Can you work these out from the drawing? Everything is in mm from the part's minimum corner. A direction names the side the tool comes from. Coordinates: 2 decimals unless noted, no trailing zeros. Order: outer loops, then holes, each group sorted by start corner. A loop starts at its lowest first (then second) coordinate and runs counter-clockwise, first axis right, second up. Notation, with made-up numbers: (-37.5, 69.5) -> (-22.5, 69.5) arc R7 cw to (-22.5, 78.5) -> close; hole circle Ø8 at (64.5, 50). An arc over 180 degrees is marked (long way). Return JSON: item names as keys, results as strings. Group by question number.
1) If we section it at A-A, the plane z = 19.5: Please give me the cut outline in (x, y).
2) For the marked faces 1 and 2, which set-ups out of +Z, -Z, +X, -X, +Y, -Y let a thin tool reach every point of the face, with its end or its side?
3) If we section it at B-B, the plane y = 12.25: Please give me the cut outline in (x, z), then the cut area to 3 significant figures.
4) For pin 1 (7.5 mm diameter, centred on x = 29, y = 8.5, fed in from +Z), with a flat end and sliding along its axis, tell me the tip position at first contact or that it passes through.
5) Thinking about a two-plate mould opening in X: for the marked faces 3, 4 and 5, which applies, +X half, -X half, draft (parallel to the pull), parting line (faces both ways), or undercut?
6) If I drill on probe 1 along X at (y, z) = (15.5, 20.5); probe 2 along Z at (x, y) = (9, 20.75), over which ranges is the centre line in solid material (lowest first)? Write a range as from..to.
7) If we section it at C-C, the plane x = 32: Please give me the cut outline in (y, z), then the cut area to 3 significant figures.
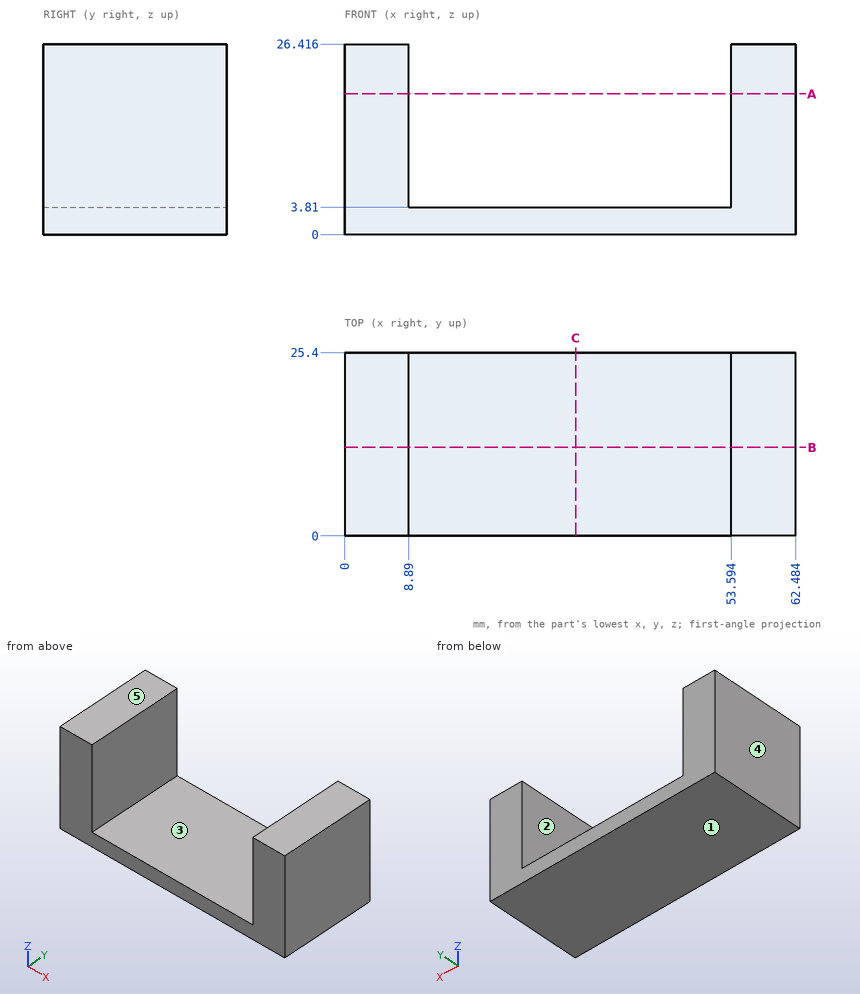
Result sheet:
{
 "1": {"outline": "(0, 0) -> (8.89, 0) -> (8.89, 25.4) -> (0, 25.4) -> close; (53.59, 0) -> (62.48, 0) -> (62.48, 25.4) -> (53.59, 25.4) -> close"},
 "2": {"face 1": "-Z, +X, -X, +Y, -Y", "face 2": "+Z, +Y, -Y"},
 "3": {"outline": "(0, 0) -> (62.48, 0) -> (62.48, 26.42) -> (53.59, 26.42) -> (53.59, 3.81) -> (8.89, 3.81) -> (8.89, 26.42) -> (0, 26.42) -> close", "area": "640 mm2"},
 "4": {"pin 1": "stops at z = 3.81"},
 "5": {"face 3": "undercut", "face 4": "-X half", "face 5": "draft"},
 "6": {"probe 1": "x = 0..8.89, 53.59..62.48", "probe 2": "z = 0..3.81"},
 "7": {"outline": "(0, 0) -> (25.4, 0) -> (25.4, 3.81) -> (0, 3.81) -> close", "area": "96.8 mm2"}
}
